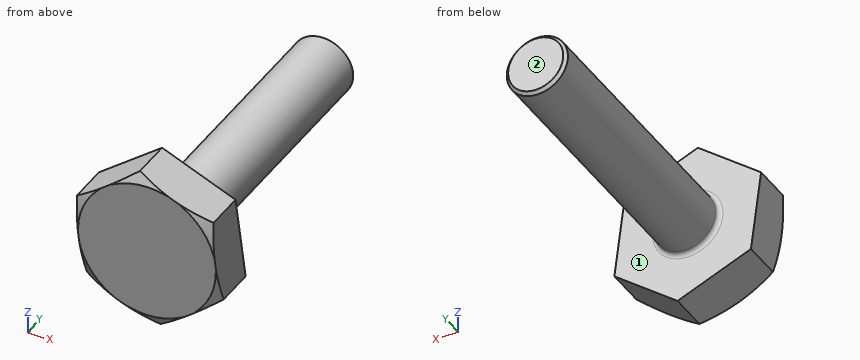
from build123d import *

# Parameters (mm, degrees)
BOSS_EXTRUDE2_DEPTH = 1.5
SKETCH3_OUTSIDE_W   = 13.432
SKETCH3_OUTSIDE_H   = 13.79
SKETCH3_OUTSIDE_R   = 2.25
CUT_EXTRUDE2_DEPTH  = 1.5
CUT_EXTRUDE2_DRAFT  = 60
SKETCH4_R           = 1
BOSS_EXTRUDE3_DEPTH = 9
CHAMFER1_SIZE       = 0.1
FILLET1_R           = 0.15


with BuildPart() as part:
    # Sketch1 → Boss-Extrude2 (new body)
    with BuildSketch(Plane(origin=(0, 0, 0), x_dir=(1, 0, 0), z_dir=(0, 1, 0))):
        Polygon((2.065411664, -1.576094749), (2.397643923, 1.000651596), (0.332232259, 2.576746345), (-2.065411664, 1.576094749), (-2.397643923, -1.000651596), (-0.332232259, -2.576746345), align=None)
    extrude(amount=BOSS_EXTRUDE2_DEPTH)


with BuildPart() as cut_extrude2_tool:
    # Sketch3 outside → Cut-Extrude2 (with draft: the straight prism first)
    with BuildSketch(Plane(origin=(0, 0, 0), x_dir=(1, 0, 0), z_dir=(0, 1, 0))):
        Rectangle(SKETCH3_OUTSIDE_W, SKETCH3_OUTSIDE_H)
        Circle(SKETCH3_OUTSIDE_R, mode=Mode.SUBTRACT)
    extrude(amount=CUT_EXTRUDE2_DEPTH)
    # Cut-Extrude2: the draft: its side faces are tilted about the plane it starts from
    cut_extrude2_sides = [cut_extrude2_tool.faces().sort_by_distance(p)[0] for p in [
        (0, 0.75, 6.895),
        (6.716, 0.75, 0),
        (0, 0.75, -6.895),
        (-6.716, 0.75, 0),
        (-2.25, 0.75, 0),
    ]]
    draft(cut_extrude2_sides, Plane(origin=(0, 0, 0), x_dir=(1, 0, 0), z_dir=(0, 1, 0)), CUT_EXTRUDE2_DRAFT)


with BuildPart() as part_1:
    add(part.part)

    # Cut-Extrude2: cut by cut_extrude2_tool
    add(cut_extrude2_tool.part, mode=Mode.SUBTRACT)

    # Sketch4 → Boss-Extrude3 (add)
    with BuildSketch(Plane(origin=(0, 1.5, 0), x_dir=(1, 0, 0), z_dir=(0, 1, 0))):
        with Locations(Location((0, 0, 0), (0, 0, 270))):
            Circle(SKETCH4_R)
    extrude(amount=BOSS_EXTRUDE3_DEPTH)

    # Chamfer1
    chamfer1_edges = [part_1.edges().sort_by_distance(p)[0] for p in [
        (0, 10.5, -1),
    ]]
    chamfer(chamfer1_edges, length=CHAMFER1_SIZE)

    # Fillet1
    fillet1_edges = [part_1.edges().sort_by_distance(p)[0] for p in [
        (0, 1.5, -1),
    ]]
    fillet(fillet1_edges, radius=FILLET1_R)


solid = part_1.part
The model under review builds one solid part; all positions refer to its coordinate system, in mm. Face numbers are marked on the shaded views. A direction names the side the tool comes from. Round coordinates to 2 decimals unless told otherwise and drop trailing zeros. Loops run counter-clockwise (first coordinate to the right, second up) from the corner with the lowest first, then second, coordinate; pieces in that order, holes last. Notation, with made-up numbers: (72.25, 60) -> (112.25, 60) arc R10 ccw to (112.25, 68) -> close; hole circle Ø3 at (71.5, 80). An arc over 180 degrees is marked (long way). One line per question, with ' | ' between items. Start each with the question number.
Item 1: Wall thickness on line 1 along Y through (x, z) = (0.1, -1.75); line 2 along X through (y, z) = (5.25, 0.55); line 3 along Z through (x, y) = (0.05, 0.5): over which ranges is each line inside the solid? List them lowest first. Write a range as [from, to].
Item 2: Machinability: for the marked faces 1 and 2, which of the approach directions +Z, -Z, +X, -X, +Y, -Y give a long, thin tool a straight path to every point of the face, cutting with its end or side? Answer none if there is none.
Item 3: Add section B-B, the plane x = 0. Write out the cut boundary in (y, z), then the cut area to 3 significant figures.
Item 4: For pin 1 (2 mm diameter, centred on x = -0.5, y = 6.5, fed in from -Z); pin 2 (2 mm diameter, centred on x = -1.5, y = 1.5, fed in from -Z); pin 3 (1 mm diameter, centred on y = 3, z = -1, fed in from +X), all flat-tipped, find the tip position at first contact; note any pin that passes through.
Item 5: Add section C-C, the plane y = 8. Write out the cut boundary in (x, z).
Return value:
1) line 1: y = [0, 1.5] | line 2: x = [-0.84, 0.84] | line 3: z = [-2.46, 2.42]
2) face 1: +Y | face 2: +Z, -Z, +X, -X, +Y
3) outline: (0, -2.25) -> (0.11, -2.44) -> (1.5, -2.44) -> (1.5, -1.15) arc R0.15 cw to (1.65, -1) -> (10.4, -1) -> (10.5, -0.9) -> (10.5, 0.9) -> (10.4, 1) -> (1.65, 1) arc R0.15 cw to (1.5, 1.15) -> (1.5, 2.44) -> (0.11, 2.44) -> (0, 2.25) -> close | area: 25.3 mm2
4) pin 1: stops at z = -1 | pin 2: stops at z = -2.23 | pin 3: stops at x = 0.87
5) outline: circle Ø2 at (0, 0)
